Autodesk Inventor part; units mm, degrees
ref_plane "Pracovní rovina1" through (16, 0, 0) normal (1, 0, 0) x (0, 1, 0)
ref_plane "XZ Plane" through (0, 0, 0) normal (0, 1, 0) x (-1, 0, 0)
ref_plane "XY Plane" through (0, 0, 0) normal (0, 0, 1) x (1, 0, 0)
sketch "Náčrt3" plane through (0, 0, 0) normal (1, 0, 0) x (0, 1, 0)
  line L0 (0, 0) -> (0, 16)
  line L1 (0, 16) -> (21, 16)
  line L2 (21, 16) -> (21, 14.5)
  line L3 (21, 14.5) -> (22.5, 14.5)
  line L4 (22.5, 14.5) -> (22.5, 16)
  line L5 (22.5, 16) -> (25.5, 16)
  line L6 (25.5, 16) -> (25.5, 14.5)
  line L7 (25.5, 14.5) -> (27, 14.5)
  line L8 (27, 14.5) -> (27, 16)
  line L9 (27, 16) -> (29.2548, 16)
  line L10 (32, 0) -> (0, 0)
  arc A0 (32, 0) -> (29.2548, 16) centre (-16, 0) ccw
  dimension "d4" = 16
  dimension "d5" = 21
  dimension "d6" = 3
  dimension "d7" = 1.5
  dimension "d8" = 1.5
  dimension "d9" = 14.5
  dimension "d12" = 96
  dimension "d13" = 32
revolve "Rotace1" add sketch "Náčrt3" angle 360 about axis through (0, 32, 0) along (0, -1, 0)
sketch "Náčrt4" plane through (0, 0, 0) normal (1, 0, 0) x (0, 1, 0)
  line L0 (0, 16) -> (0, -16)
  line L1 (0, 13) -> (10, 13)
  line L2 (10, 13) -> (10, 10)
  line L3 (20.5263, 0) -> (0, 0)
  line L4 (10, 10) -> (24, 10)
  line L5 (24, 10) -> (24, 0)
  line L6 (24, 0) -> (20.5263, 0)
  line L7 (-6.4, 0) -> (38.4, 0)
  dimension "d14" = 10
  dimension "d15" = 13
  dimension "d16" = 10
  dimension "d17" = 24
revolve "Rotace2" cut sketch "Náčrt4" angle 360 about axis through (0, -10, 0) along (0, 1, 0)
fillet "Zaoblení1" radius 2 2 edges at (0, 10, -13) (0, 24, -10)
ref_plane "Pracovní rovina1" through (16, 0, 0) normal (1, 0, 0) x (0, 1, 0)
sketch "Náčrt5" plane through (16, 0, 0) normal (1, 0, 0) x (0, 1, 0)
  line L0 (-6.4, 0) -> (38.4, 0)
  line L1 (0, -22.4) -> (0, 22.4)
  point P0 (0, 0)
  point P1 (16, 0)
  dimension "d21" = 16
hole "Díra1" at (16, 16, 0) direction (-1, 0, 0) diameter 5 end through all
properties part number "Piston_head" material "Ocel"
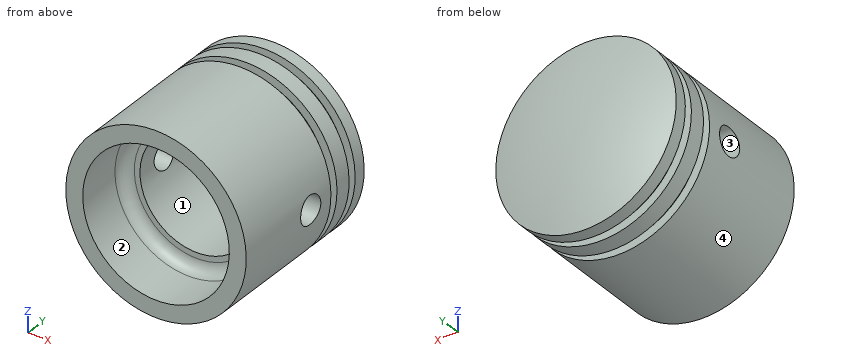
Part model, mm, in its own coordinate system. Face numbers are marked on the shaded views. Round coordinates to 2 decimals unless told otherwise and drop trailing zeros. Loops run counter-clockwise (first coordinate to the right, second up) from the corner with the lowest first, then second, coordinate; pieces in that order, holes last. Notation, with made-up numbers: (14, 86.25) - (55, 86.25) arc R31 ccw to (55, 113.25) - close; hole circle Ø10 at (80.25, 84.5). An arc over 180 degrees is marked (long way). Answer as a JSON object with one key per item and string values.
Item 1: Pin check, flat tips, straight feed: pin 1 (1.5 mm diameter, centred on x = -8, y = 21, fed in from +Z); pin 2 (10 mm diameter, centred on y = 4, z = -11, fed in from +X); pin 3 (2 mm diameter, centred on x = 2.5, z = -1, fed in from +Y); pin 4 (3 mm diameter, centred on y = 16, z = 0, fed in from +X). Stop position of each tip, or through.
Output:
{"pin 1": "z = 14.26", "pin 2": "x = 14.83", "pin 3": "y = 31.97", "pin 4": "through"}
Item 2: Wall check: L1, parallel to X at y = 4.5, z = 0; L2, parallel to Y at x = 10, z = -11.5; L3, parallel to X at y = 3.5, z = -10.5. Give the ranges that are in metal, low to high.
Output:
{"L1": "-16 to -13, 13 to 16", "L2": "0 to 21, 22.5 to 25.5, 27 to 29.52", "L3": "-12.07 to -7.66, 7.66 to 12.07"}
Item 3: Band-saw the part on A-A on y = 15. List the corners of the cut face in (x, z).
Output:
{"outline": "(-15.84, -2.29) arc R16 ccw to (15.84, -2.29) - (9.73, -2.29) arc R10 cw to (-9.73, -2.29) - close; (-15.84, 2.29) - (-9.73, 2.29) arc R10 cw to (9.73, 2.29) - (15.84, 2.29) arc R16 ccw to start"}
Item 4: Band-saw the part on C-C on y = 9. List the corners of the cut face in (x, z), plus the area to 3 significant figures.
Output:
{"outline": "circle Ø32 at (0, 0); hole circle Ø25.46 at (0, 0)", "area": "295 mm2"}
Item 5: Pull direction X, two halves, no side cores. Call the marked faces 1, 2, 3 and 4: pulls with the +X half, pulls with the -X half, needs draft (parallel to the pull), parting line crosses it, or undercut.
Output:
{"face 1": "undercut", "face 2": "undercut", "face 3": "needs draft", "face 4": "parting line crosses it"}
Item 6: Band-saw the part on B-B on z = 1.5. State how many separate pieces and enclosed holes the cut face has, plus the area to 3 significant figures.
Output:
{"separate pieces": "3", "enclosed holes": "0", "area": "401 mm2"}
